Job drawing, mm, ordinate dimensions from the low corner. One solid piece. A direction names the side the tool comes from. Round coordinates to 2 decimals unless told otherwise and drop trailing zeros. Loops run counter-clockwise (first coordinate to the right, second up) from the corner with the lowest first, then second, coordinate; pieces in that order, holes last.
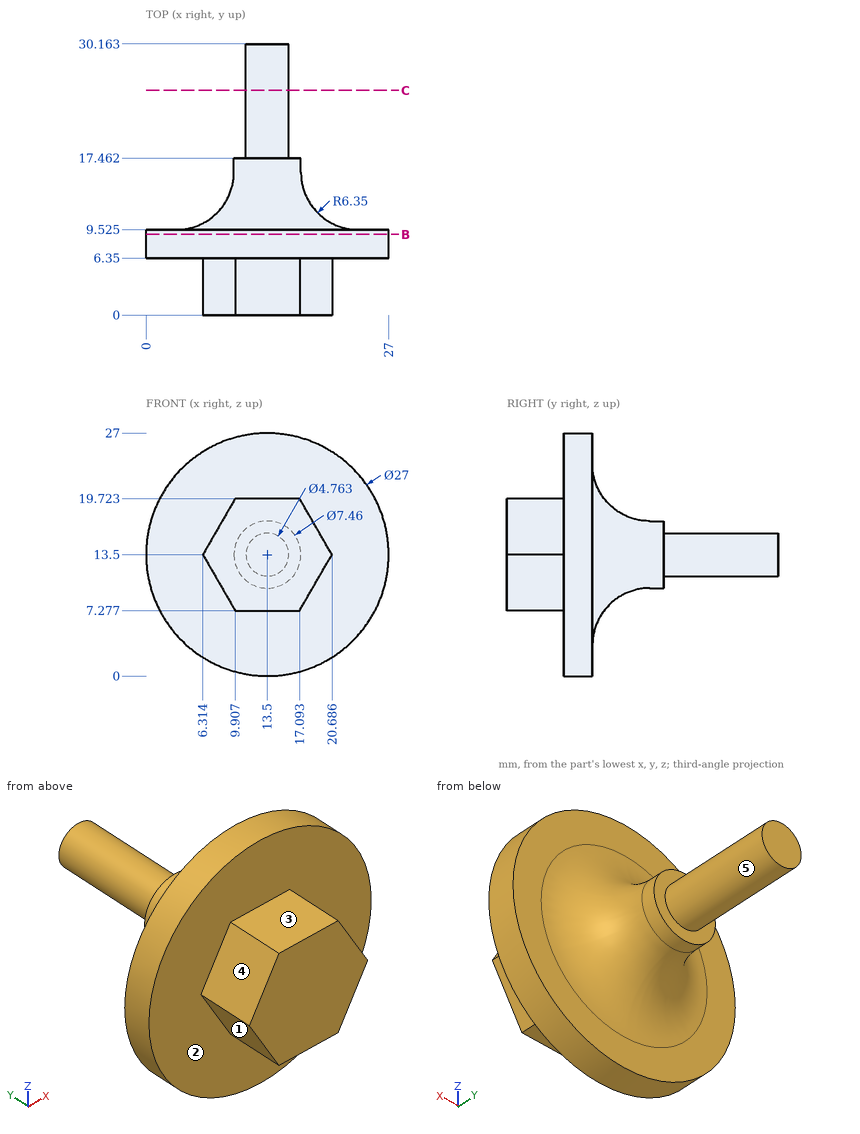
(1) Slice it at C-C on y = 25. List the corners of the cut face in (x, z).
Responses:
outline: circle Ø4.76 at (13.5, 13.5)
(2) Slice it at B-B on y = 9. List the corners of the cut face in (x, z).
Responses:
outline: circle Ø27 at (13.5, 13.5)
(3) Which spindle directions (+Z, -Z, +X, -X, +Y, -Y) get a long thin tool onto all of the face, cutting with end or side? Do the marked faces 1, 2, 3, 4 and 5. Say none if no direction does.
Responses:
face 1: -Z, -X, -Y
face 2: -Y
face 3: +Z, +X, -X, -Y
face 4: +Z, -X, -Y
face 5: +Y
(4) Probe line 1 (Y direction, x = 19.25, z = 19.5); line 2 (Z direction, x = 16, y = 5.5); line 3 (Y direction, x = 16.25, z = 22.25). List the from-to ranges inside material, lowest first.
Responses:
line 1: y = 6.35 to 9.78
line 2: z = 7.28 to 19.72
line 3: y = 6.35 to 9.59
(5) Pin check, flat tips, straight feed: P1, Ø10, axis at x = 16, y = 25, coming from the -Z side; P2, Ø5, axis at x = 23, z = 11, coming from the +Y side (1 decimal); P3, Ø1.5, axis at x = 4.5, z = 13, coming from the +Y side. Stop position of each tip, or through.
Responses:
P1: stops at z = 11.12
P2: stops at y = 10.2
P3: stops at y = 9.79
